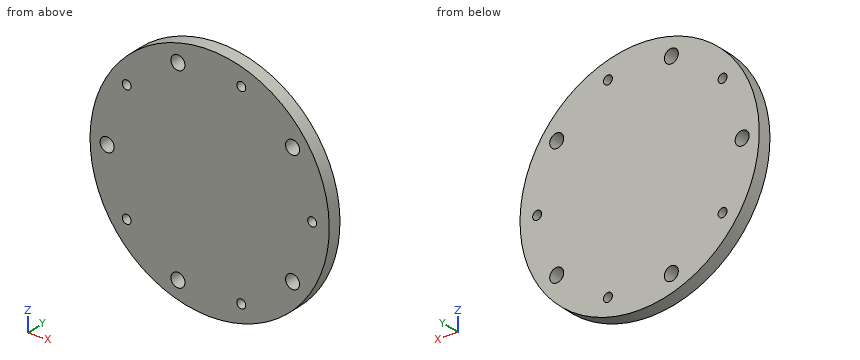
from build123d import *

# Parameters (mm, degrees)
SKETCH19_R          = 70
BOSS_EXTRUDE2_DEPTH = 8
SKETCH19_3_R        = 4.1
SKETCH19_3_R_2      = 2.6
BOLT_HOLES_DEPTH    = 8
CIRPATTERN10_COUNT  = 5


with BuildPart() as part:
    # Sketch1 → Revolve1 (revolve)
    with BuildSketch(Plane.XY, mode=Mode.PRIVATE) as revolve1_sk:
        Polygon((-47.4, 0), (-47.4, -8), (-17.4, -8), (-7, -8), (0, -8), (0, 0), align=None)
    revolve(revolve1_sk.sketch.rotate(Axis((0, -8, 0), (0, 1, 0)), 180), axis=Axis((0, -8, 0), (0, 1, 0)))

    # Sketch19 → Boss-Extrude2 (add)
    with BuildSketch(Plane.XZ.offset(8)):
        with Locations(Location((0, 0, 0), (0, 0, 270))):
            Circle(SKETCH19_R)
    extrude(amount=-BOSS_EXTRUDE2_DEPTH)

    # Sketch19<3> → Bolt holes (cut)
    with BuildSketch(Plane.XZ.offset(8)):
        with Locations(Location((-60, 0, 0), (0, 0, 270))):
            Circle(SKETCH19_3_R)
        with Locations(Location((-48.541019662, -35.267115138, 0), (0, 0, 270))):
            Circle(SKETCH19_3_R_2)
    bolt_holes = extrude(amount=-BOLT_HOLES_DEPTH, mode=Mode.SUBTRACT)

    # CirPattern10: Bolt holes ×5 about axis
    cirpattern10_axis = Axis((0, 0, 0), (0, 1, 0))
    for i in range(1, CIRPATTERN10_COUNT):
        add(bolt_holes.rotate(cirpattern10_axis, i * 360 / CIRPATTERN10_COUNT), mode=Mode.SUBTRACT)


solid = part.part
Input: part model. Units: mm. Frame: model coordinates. Coordinates: 2 decimals unless noted, no trailing zeros. Write each loop counter-clockwise with the first axis right and the second up, starting at its lowest first coordinate (ties: lowest second). Pieces come first, ordered by that corner, then holes. Notation, with made-up numbers: M -39.75,18.5 L -17.75,18.5 A33 ccw -17.75,55.5 Z; hole C -39,75.5 d8. An arc over 180 degrees is marked long. Answer as a JSON object with one key per item and string values. Group by question number.
(1) Ray query, line 1 along X through (y, z) = (-7.5, -55); line 2 along Z through (x, y) = (46.5, -2.25); line 3 along X through (y, z) = (-6.75, -57.5). Return the intervals inside material, ascending. Write a range as [from, to].
(2) Section A-A on z = 0. Output: boundary loops of the cut face in (x, y), plus the area to 3 significant figures.
(3) Section B-B on x = -60. Output: boundary loops of the cut face in (y, z).
(4) Section C-C on y = -6. Give the number of separate pieces and of enclosed holes in the cut face, plus the area to 3 significant figures.
(5) Section D-D on z = -16. Output: boundary loops of the cut face in (x, y), plus the area to 3 significant figures.
(6) Contact query for flat-ended pins moving along their axis: P1, Ø13, axis at x = 48.54, z = -35.27, coming from the +Y side; P2, Ø4, axis at x = -51.5, y = -3, coming from the +Z side; P3, Ø4.5, axis at x = -48.54, z = -35.27, coming from the -Y side; P4, Ø1, axis at y = -3, z = 10.5, coming from the -X side. Output: stop coordinate, or through.
Result set:
{
 "1": {"line 1": "x = [-43.3, -22.08], [-15, 16.96], [20.12, 43.3]", "line 2": "z = [-52.32, -38.82], [-31.71, 31.71], [38.82, 52.32]", "line 3": "x = [-39.92, -22.62], [-14.46, 15.98], [21.1, 39.92]"},
 "2": {"outline": "M -70,-8 L -64.1,-8 L -64.1,0 L -70,0 Z; M -55.9,-8 L 57.4,-8 L 57.4,0 L -55.9,0 Z; M 62.6,-8 L 70,-8 L 70,0 L 62.6,0 Z", "area": "1,010 mm2"},
 "3": {"outline": "M -8,-36.06 L 0,-36.06 L 0,-4.1 L -8,-4.1 Z; M -8,4.1 L 0,4.1 L 0,36.06 L -8,36.06 Z"},
 "4": {"separate pieces": "1", "enclosed holes": "10", "area": "15,000 mm2"},
 "5": {"outline": "M -68.15,-8 L 68.15,-8 L 68.15,0 L -68.15,0 Z", "area": "1,090 mm2"},
 "6": {"P1": "stops at y = 0", "P2": "stops at z = 49.49", "P3": "passes through", "P4": "stops at x = -69.28"}
}
